```python
from build123d import *

# Parameters (mm, degrees)
F1_DEPTH      = 12.7
F1_DEPTH_BACK = 12.7
F2_W          = 11.756946
F2_H          = 25.4
F3_DEPTH      = 2.54
F4_W          = 25.4
F4_H          = 25.4
F5_DEPTH      = 6.35


with BuildPart() as f1:
    # F0 (on Front) → F1 (new body, two sides)
    with BuildSketch(Plane.XZ) as f1_sk:
        Polygon((-5.878473, 6.096), (-9.398, 0), (9.398, 0), (5.878473, 6.096), align=None)
    extrude(amount=F1_DEPTH)
    extrude(f1_sk.sketch, amount=-F1_DEPTH_BACK)

    # F2 (on face) → F3 (join)
    with BuildSketch(Plane.XY.offset(6.096)):
        Rectangle(F2_W, F2_H)
    extrude(amount=F3_DEPTH)

    # F4 (on face) → F5 (join)
    with BuildSketch(Plane.XY.offset(8.636)):
        Rectangle(F4_W, F4_H)
    extrude(amount=F5_DEPTH)


solid = f1.part
```
Design review of the part built by this model. Coordinates are the model's own, in mm. A direction names the side the tool comes from. Round coordinates to 2 decimals unless told otherwise and drop trailing zeros. Write each loop counter-clockwise with the first axis right and the second up, starting at its lowest first coordinate (ties: lowest second). Pieces come first, ordered by that corner, then holes. Notation, with made-up numbers: (18, 88.5) -> (46, 88.5) arc R24 cw to (46, 101.5) -> close; hole circle Ø8 at (54.25, -39). An arc over 180 degrees is marked (long way). Answer in a Markdown table with one row per item.
Q1. Take a section at A-A, the plane y = -3.75. State the section outline as (x, z) points.
The answers:
| item | result |
|---|---|
| outline | (-12.7, 8.64) -> (-5.88, 8.64) -> (-5.88, 6.1) -> (-9.4, 0) -> (9.4, 0) -> (5.88, 6.1) -> (5.88, 8.64) -> (12.7, 8.64) -> (12.7, 14.99) -> (-12.7, 14.99) -> close |
Q2. To check wall thickness, follow L1, parallel to Z at x = 6, y = 9.5; L2, parallel to Z at x = -10.5, y = 7.25; L3, parallel to Z at x = 9, y = -6. State the ranges of each line that lie inside material, in increasing order. Write a range as [from, to].
The answers:
| item | result |
|---|---|
| L1 | [0, 5.89], [8.64, 14.99] |
| L2 | [8.64, 14.99] |
| L3 | [0, 0.69], [8.64, 14.99] |
Q3. For faces 5 (the face through (-5.878, 0, 7)), 6 (the face through (5.878, 0, 7)), 7 (the face through (12.7, 0, 12)), list the 3-axis set-ups (+Z, -Z, +X, -X, +Y, -Y) from which the entire face can be reached by the end or side of a thin tool; tool diameter is ignored.
The answers:
| item | result |
|---|---|
| face 5 | -X, +Y, -Y |
| face 6 | +X, +Y, -Y |
| face 7 | +Z, -Z, +X, +Y, -Y |
Q4. Draft analysis for pull direction Z (two halves, no side actions). For faces 1 (the face through (9, 0, 8.636)), 2 (the face through (0, 0, 14.986)), 3 (the face through (0, 0, 0)), 4 (the face through (-12.7, 0, 12)), state which applies: +Z half, -Z half, draft (parallel to the pull), parting line (faces both ways), or undercut.
The answers:
| item | result |
|---|---|
| face 1 | undercut |
| face 2 | +Z half |
| face 3 | -Z half |
| face 4 | draft |
Q5. Take a section at B-B, the plane z = 7.5. State the section outline as (x, y) points.
The answers:
| item | result |
|---|---|
| outline | (-5.88, -12.7) -> (5.88, -12.7) -> (5.88, 12.7) -> (-5.88, 12.7) -> close |
Q6. Take a section at C-C, the plane x = 11.25. State the section outline as (y, z) points, then the cut area to 3 significant figures.
The answers:
| item | result |
|---|---|
| outline | (-12.7, 8.64) -> (12.7, 8.64) -> (12.7, 14.99) -> (-12.7, 14.99) -> close |
| area | 161 mm² |
